from build123d import *

# Parameters (mm, degrees)
SKETCH2_W            = 55
SKETCH2_H            = 5
SKETCH2_W_2          = 5
BOSS_EXTRUDE3_DEPTH  = 20
SKETCH3_W            = 5
SKETCH3_H            = 5
CUT_EXTRUDE1_DEPTH   = 10
SKETCH5_W            = 5
SKETCH5_H            = 5
CUT_EXTRUDE2_DEPTH   = 10
SKETCH6_W            = 5
SKETCH6_H            = 5
CUT_EXTRUDE3_DEPTH   = 10
SKETCH7_R            = 1
CUT_EXTRUDE5_DEPTH   = 10
SKETCH8_R            = 1
CUT_EXTRUDE6_DEPTH   = 10
SKETCH9_R            = 1
CUT_EXTRUDE7_DEPTH   = 10
SKETCH10_R           = 1
CUT_EXTRUDE8_DEPTH   = 10
SKETCH11_W           = 55
SKETCH11_H           = 41
BOSS_EXTRUDE10_DEPTH = 5
SKETCH12_R           = 1
CUT_EXTRUDE9_DEPTH   = 10
SKETCH13_R           = 1
CUT_EXTRUDE10_DEPTH  = 10
SKETCH14_R           = 1
CUT_EXTRUDE11_DEPTH  = 10
SKETCH15_R           = 1
CUT_EXTRUDE12_DEPTH  = 10


with BuildPart() as part:
    # Sketch2 → Boss-Extrude3 (new body)
    with BuildSketch(Plane(origin=(0, 0, 0), x_dir=(1, 0, 0), z_dir=(0, 1, 0))):
        with Locations((-27.5, 2.5)):
            Rectangle(SKETCH2_W, SKETCH2_H)
        Polygon((-5, 5), (0, 5), (0, 41), (-5, 41), (-5, 36), (-5, 30.997910325), (-5, 10), align=None)
        Polygon((-5, 36), (-5, 41), (-50, 41), (-50, 36), (-45, 36), (-10.013652048, 36), (-9.330274009, 36), align=None)
        Polygon((-55, 41), (-55, 5), (-50, 5), (-50, 10), (-50, 31), (-50, 36), (-50, 41), align=None)
        with Locations((-47.5, 33.5)):
            Rectangle(SKETCH2_W_2, SKETCH2_H)
        with Locations((-47.5, 7.5)):
            Rectangle(SKETCH2_W_2, SKETCH2_H)
        Polygon((-10.013652048, 30.997910325), (-5, 30.997910325), (-5, 36), (-9.330274009, 36), (-10.013652048, 36), align=None)
        with Locations((-7.5, 7.5)):
            Rectangle(SKETCH2_W_2, SKETCH2_H)
    extrude(amount=BOSS_EXTRUDE3_DEPTH)

    # Sketch3 → Cut-Extrude1 (cut)
    with BuildSketch(Plane(origin=(0, 20, 0), x_dir=(1, 0, 0), z_dir=(0, 1, 0))):
        with Locations((-7.513652048, 33.497910325)):
            Rectangle(SKETCH3_W, SKETCH3_H)
    extrude(amount=-CUT_EXTRUDE1_DEPTH, mode=Mode.SUBTRACT)

    # Sketch5 → Cut-Extrude2 (cut)
    with BuildSketch(Plane(origin=(0, 20, 0), x_dir=(1, 0, 0), z_dir=(0, 1, 0))):
        with Locations((-47.5, 33.5)):
            Rectangle(SKETCH5_W, SKETCH5_H)
    extrude(amount=-CUT_EXTRUDE2_DEPTH, mode=Mode.SUBTRACT)

    # Sketch6 → Cut-Extrude3 (cut)
    with BuildSketch(Plane(origin=(0, 20, 0), x_dir=(1, 0, 0), z_dir=(0, 1, 0))):
        with Locations((-47.5, 7.5)):
            Rectangle(SKETCH6_W, SKETCH6_H)
        with Locations((-7.5, 7.5)):
            Rectangle(SKETCH6_W, SKETCH6_H)
    extrude(amount=-CUT_EXTRUDE3_DEPTH, mode=Mode.SUBTRACT)

    # Sketch7 → Cut-Extrude5 (cut)
    with BuildSketch(Plane(origin=(0, 10, 0), x_dir=(1, 0, 0), z_dir=(0, 1, 0))):
        with Locations(Location((-47.5, 33.5, 0), (0, 0, 270))):
            Circle(SKETCH7_R)
    extrude(amount=-CUT_EXTRUDE5_DEPTH, mode=Mode.SUBTRACT)

    # Sketch8 → Cut-Extrude6 (cut)
    with BuildSketch(Plane(origin=(0, 10, 0), x_dir=(1, 0, 0), z_dir=(0, 1, 0))):
        with Locations(Location((-7.513652048, 33.497910325, 0), (0, 0, 270))):
            Circle(SKETCH8_R)
    extrude(amount=-CUT_EXTRUDE6_DEPTH, mode=Mode.SUBTRACT)

    # Sketch9 → Cut-Extrude7 (cut)
    with BuildSketch(Plane(origin=(0, 10, 0), x_dir=(1, 0, 0), z_dir=(0, 1, 0))):
        with Locations(Location((-47.5, 7.5, 0), (0, 0, 270))):
            Circle(SKETCH9_R)
    extrude(amount=-CUT_EXTRUDE7_DEPTH, mode=Mode.SUBTRACT)

    # Sketch10 → Cut-Extrude8 (cut)
    with BuildSketch(Plane(origin=(0, 10, 0), x_dir=(1, 0, 0), z_dir=(0, 1, 0))):
        with Locations(Location((-7.5, 7.5, 0), (0, 0, 270))):
            Circle(SKETCH10_R)
    extrude(amount=-CUT_EXTRUDE8_DEPTH, mode=Mode.SUBTRACT)

    # Sketch11 → Boss-Extrude10 (add)
    with BuildSketch(Plane(origin=(0, 0, 0), x_dir=(-1, 0, 0), z_dir=(0, -1, 0))):
        with Locations((27.5, 20.5)):
            Rectangle(SKETCH11_W, SKETCH11_H)
    extrude(amount=BOSS_EXTRUDE10_DEPTH)

    # Sketch12 → Cut-Extrude9 (cut)
    with BuildSketch(Plane(origin=(0, 20, 0), x_dir=(1, 0, 0), z_dir=(0, 1, 0))):
        with Locations(Location((-52.5, 38.5, 0), (0, 0, 270))):
            Circle(SKETCH12_R)
    extrude(amount=-CUT_EXTRUDE9_DEPTH, mode=Mode.SUBTRACT)

    # Sketch13 → Cut-Extrude10 (cut)
    with BuildSketch(Plane(origin=(0, 20, 0), x_dir=(1, 0, 0), z_dir=(0, 1, 0))):
        with Locations(Location((-2.506826024, 38.498955163, 0), (0, 0, 270))):
            Circle(SKETCH13_R)
    extrude(amount=-CUT_EXTRUDE10_DEPTH, mode=Mode.SUBTRACT)

    # Sketch14 → Cut-Extrude11 (cut)
    with BuildSketch(Plane(origin=(0, 20, 0), x_dir=(1, 0, 0), z_dir=(0, 1, 0))):
        with Locations(Location((-52.5, 2.5, 0), (0, 0, 270))):
            Circle(SKETCH14_R)
    extrude(amount=-CUT_EXTRUDE11_DEPTH, mode=Mode.SUBTRACT)

    # Sketch15 → Cut-Extrude12 (cut)
    with BuildSketch(Plane(origin=(0, 20, 0), x_dir=(1, 0, 0), z_dir=(0, 1, 0))):
        with Locations(Location((-2.5, 2.5, 0), (0, 0, 270))):
            Circle(SKETCH15_R)
    extrude(amount=-CUT_EXTRUDE12_DEPTH, mode=Mode.SUBTRACT)


solid = part.part
Read the model definition and answer for the solid it produces. Units are mm, in the model's axes. A direction names the side the tool comes from. Round coordinates to 2 decimals unless told otherwise and drop trailing zeros. Loops run counter-clockwise (first coordinate to the right, second up) from the corner with the lowest first, then second, coordinate; pieces in that order, holes last.
Q1. Section C-C on x = -37 is taken. Write down the section's boundary in (y, z).
Q2. Determine the mould class of faces 1 (the face through (-55, 8, -20)), 2 (the face through (-27, 8, 0)), 3 (the face through (-2, 10, -39)), 4 (the face through (-27, 8, -41)) for opening direction Z: released by +Z, released by -Z, zero draft, split by the parting line, or undercut.
Q3. Section B-B on y = 16.75 is taken. Give the number of separate pieces and of enclosed holes in the cut face, and give its area (3 significant figures).
Q4. Which of the six approach directions +Z, -Z, +X, -X, +Y, -Y give full straight-line access (tool end or side, diameter ignored) to faces 5 (the face through (-27, -5, -21)), 6 (the face through (-49, 10, -8))?
Q5. Each of these flat-tipped pins is pushed along its axis until it touches: pin 1 (1.8 mm diameter, centred on x = -2.51, z = -38.5, fed in from +Y); pin 2 (0.6 mm diameter, centred on x = -7.5, z = -8, fed in from +Y). Where does it stop, or does it pass through?
Q6. Consider probe 1 along X at (y, z) = (12.75, -38.5); probe 2 along Z at (x, y) = (-5.5, 2); probe 3 along X at (y, z) = (11.25, -32.5). Determine where each line is inside the solid, lowest interval first.
Q7. Section A-A on z = -14 is taken. Write down the section's boundary in (x, y).
Q8. Section D-D on z = -7.5 is taken. Write down the section's boundary in (x, y), and give its area (3 significant figures).
Output:
1. outline: (-5, -41) - (20, -41) - (20, -36) - (0, -36) - (0, -5) - (20, -5) - (20, 0) - (-5, 0) - close
2. face 1: zero draft
2. face 2: released by +Z
2. face 3: undercut
2. face 4: released by -Z
3. separate pieces: 1
3. enclosed holes: 5
3. area: 848 mm2
4. face 5: +Z, -Z, +X, -X, -Y
4. face 6: +Y
5. pin 1: stops at y = 10
5. pin 2: stops at y = 0
6. probe 1: x = -55 to -53.5, -51.5 to -3.51, -1.51 to 0
6. probe 2: z = -41 to -31, -10 to 0
6. probe 3: x = -55 to -50, -5.01 to 0
7. outline: (-55, -5) - (0, -5) - (0, 20) - (-5, 20) - (-5, 0) - (-50, 0) - (-50, 20) - (-55, 20) - close
8. outline: (-55, -5) - (0, -5) - (0, 20) - (-5, 20) - (-5, 10) - (-6.5, 10) - (-6.5, 0) - (-8.5, 0) - (-8.5, 10) - (-10, 10) - (-10, 0) - (-45, 0) - (-45, 10) - (-46.5, 10) - (-46.5, 0) - (-48.5, 0) - (-48.5, 10) - (-50, 10) - (-50, 20) - (-55, 20) - close
8. area: 535 mm2
